```python
from build123d import *

# Parameters (mm, degrees)
F0_W     = 80
F0_H     = 140
F1_DEPTH = 10
F2_D     = 5.5
F3_D     = 5.5
F4_W     = 80
F4_H     = 20
F5_DEPTH = 10
F6_W     = 80
F6_H     = 60
F7_DEPTH = 10
F9_D     = 5.5


with BuildPart() as f1:
    # F0 (on Top) → F1 (new body)
    with BuildSketch(Plane.XY):
        Rectangle(F0_W, F0_H)
    extrude(amount=F1_DEPTH)

    # F2 (through all)
    with Locations(Plane(origin=(0, 0, 0), x_dir=(1, 0, 0), z_dir=(0, 0, -1))):
        with Locations((25, -7), (25, 13), (25, -33), (25, -53), (-12, -53), (-12, -33), (-25, -33), (-25, -53), (-12, -7), (-25, -7), (-12, 13), (-25, 13)):
            Hole(F2_D / 2)

    # F3 (through all)
    with Locations(Plane(origin=(0, 0, 0), x_dir=(1, 0, 0), z_dir=(0, 0, -1))):
        with Locations((0, -40), (0, -55), (0, 35), (0, -20)):
            Hole(F3_D / 2)

    # F4 (on face) → F5 (join)
    with BuildSketch(Plane.XY):
        with Locations((0, -60.125451535)):
            Rectangle(F4_W, F4_H)
    extrude(amount=-F5_DEPTH)

    # F6 (on face) → F7 (join)
    with BuildSketch(Plane.XY.offset(10)):
        with Locations((0, -40)):
            Rectangle(F6_W, F6_H)
    extrude(amount=F7_DEPTH)

    # F9 (through all)
    with Locations(Plane.XY.offset(20)):
        with Locations((-25, -35), (25, -35), (-25, -60), (25, -60)):
            Hole(F9_D / 2)


solid = f1.part
```
Here's how the part is built. I have some questions about the finished solid (model axes, mm). A direction names the side the tool comes from. Coordinates: 2 decimals unless noted, no trailing zeros. Loops run counter-clockwise (first coordinate to the right, second up) from the corner with the lowest first, then second, coordinate; pieces in that order, holes last. Notation, with made-up numbers: (-40, 5) - (-19, 5) arc R21 cw to (-19, 37) - close; hole circle Ø2 at (-13, -9.75). An arc over 180 degrees is marked (long way). Answer as CSV lines item,"result".
Q1. We'd pull the mould along Y, two halves only. Please class faces 1 (the face through (0.358, 17.273, 5.07)), 2 (the face through (-1, -70, 10)), 3 (the face through (-1, -50.125, -5)): pulls with the +Y half, pulls with the -Y half, needs draft (parallel to the pull), parting line crosses it, or undercut.
Response:
face 1,"undercut"
face 2,"pulls with the -Y half"
face 3,"pulls with the +Y half"
Q2. If I drill on L1, parallel to Y at x = 0, z = 4; L2, parallel to X at y = 53, z = 2.5; L3, parallel to X at y = 55, z = 4, over which ranges is the centre line in solid material (lowest first)? Write a range as [from, to].
Response:
L1,"[-70, -37.75], [-32.25, 17.25], [22.75, 37.25], [42.75, 52.25], [57.75, 70]"
L2,"[-40, -27.75], [-22.25, -14.75], [-9.25, -1.89], [1.89, 22.25], [27.75, 40]"
L3,"[-40, -26.89], [-23.11, -13.89], [-10.11, -2.75], [2.75, 23.11], [26.89, 40]"
Q3. If we section it at A-A, the plane x = 25: Give the number of separate pieces and of enclosed holes in the cut face, and give its area (4 significant figures).
Response:
separate pieces,"6"
enclosed holes,"0"
area,"1,705 mm2"
Q4. If we section it at D-D, the plane x = -31.5: Write out the boundary of the cut face in (y, z).
Response:
outline,"(-70.13, -10) - (-50.13, -10) - (-50.13, 0) - (70, 0) - (70, 10) - (-10, 10) - (-10, 20) - (-70, 20) - (-70, 0) - (-70.13, 0) - close"
Q5. For pin 1 (7 mm diameter, centred on x = 25, y = -13, fed in from -Z); pin 2 (5 mm diameter, centred on x = -17, z = 16.5, fed in from +Y), each with a flat end and sliding along its axis, tell me the tip position at first contact or that it passes through.
Response:
pin 1,"z = 0"
pin 2,"y = -10"
Q6. If we section it at B-B, the plane y = 20: Write out the boundary of the cut face in (x, z).
Response:
outline,"(-40, 0) - (-2.75, 0) - (-2.75, 10) - (-40, 10) - close; (2.75, 0) - (40, 0) - (40, 10) - (2.75, 10) - close"
Q7. For faces 4 (the face through (-1, 70, 5)), 5 (the face through (-12, -13, 10)), 6 (the face through (-1, -10, 15)), which set-ups out of +Z, -Z, +X, -X, +Y, -Y let a thin tool reach every point of the face, with its end or its side?
Response:
face 4,"+Z, -Z, +X, -X, +Y"
face 5,"-Z"
face 6,"+Z, +X, -X, +Y"
